Input: part model. Units: mm. Frame: model coordinates. A direction names the side the tool comes from. Give positions to 0.01 mm unless a question says otherwise; leave off trailing zeros. Loops run counter-clockwise (first coordinate to the right, second up) from the corner with the lowest first, then second, coordinate; pieces in that order, holes last. Notation, with made-up numbers: M 11,80.25 L 29,80.25 A29 ccw 29,107.25 Z; hole C -30,-29 d11. An arc over 180 degrees is marked long. Use a Markdown table: item, result. Add a question column.
from build123d import *

# Parameters (mm, degrees)
F1_DEPTH  = 12.7
F2_W      = 12.7
F2_H      = 12.7
F3_DEPTH  = 25.4
F5_DEPTH  = 12.7
F6_R      = 9.525
F7_DEPTH  = 6.35
F7_FACE_R = 9.525
F8_DEPTH  = 19.05
F9_R      = 6.35
F10_DEPTH = 25.4


with BuildPart() as f1:
    # F0 (on Right) → F1 (new body)
    with BuildSketch(Plane.YZ):
        Polygon((0, 19.05), (0, 0), (25.4, 0), (25.4, 19.05), (19.05, 25.4), (6.35, 25.4), align=None)
    extrude(amount=F1_DEPTH)

    # F2 (on face) → F3 (join)
    with BuildSketch(Plane.YZ.offset(12.7)):
        with Locations((12.7, 12.7)):
            Rectangle(F2_W, F2_H)
    extrude(amount=F3_DEPTH)

    # F4 (on face) → F5 (cut)
    with BuildSketch(Plane.XZ.offset(-6.35)):
        with BuildLine():
            Line((38.1, 6.35), (38.1, 19.05))
            Line((38.1, 19.05), (25.4, 19.05))
            ThreePointArc((25.4, 19.05), (22.974516, 12.7), (25.4, 6.35))
            Line((25.4, 6.35), (38.1, 6.35))
        make_face()
    extrude(amount=-F5_DEPTH, mode=Mode.SUBTRACT)



with BuildPart() as f7:
    # F6 (on face) → F7 (new body)
    with BuildSketch(Plane.XZ.offset(-6.35)):
        with Locations((32.499516, 12.7)):
            Circle(F6_R)
    extrude(amount=F7_DEPTH)


with BuildPart() as f1_1:
    add(f1.part)

    add(f7.part)  # F8 merges F7
    # F7_face (on face) → F8 (join)
    with BuildSketch(Plane(origin=(32.499516, 6.35, 12.7), x_dir=(1, 0, 0), z_dir=(0, 1, 0))):
        Circle(F7_FACE_R)
    extrude(amount=F8_DEPTH)

    # F9 (on face) → F10 (cut)
    with BuildSketch(Plane(origin=(0, 25.4, 0), x_dir=(-1, 0, 0), z_dir=(0, 1, 0))):
        with Locations((-32.499516, 12.7)):
            Circle(F9_R)
    extrude(amount=-F10_DEPTH, mode=Mode.SUBTRACT)


solid = f1_1.part
1) Section query A-A, the plane z = 12.7. Return the cut outline in (x, y), and give its area (3 significant figures).
2) Pull-direction query (X, two-part tool) for faces 1 (the flat face through (6.26, 22.27, 22.18)), 2 (the flat face through (0, 13, 13)), 3 (the cylindrical face through (41.585, 12.522, 9.839)); classes: pulls with the +X half, pulls with the -X half, needs draft (parallel to the pull), parting line crosses it, or undercut.
3) Section query B-B, the plane y = 24. Return the cut outline in (x, z) (3 decimals).
4) Ray query, line 1 (X direction, y = 20, z = 12.25); line 2 (Y direction, x = 19.5, z = 9). Return the intervals inside material, ascending. Write a range as [from, to].
5) Section query C-C, the plane x = 34.5. Return the cut outline in (y, z), and give its area (3 significant figures).
6) Section query D-D, the plane y = 8.75. Return the cut outline in (x, z) (3 decimals), and give its area (3 significant figures).
7) Contact query for flat-ended pins moving along their axis: P1, Ø8, axis at x = 18, z = 6.5, coming from the -Y side; P2, Ø6, axis at y = 3, z = 22, coming from the +X side; P3, Ø3, axis at x = 14.5, z = 3.5, coming from the -Y side; P4, Ø5, axis at x = 32, y = 18, coming from the -Z side (3 decimals). Output: stop coordinate, or through.
8) Reachability of faces 4 (the flat face through (19, 13, 19.05)), 5 (the flat face through (6.26, 3.22, 22.27)), 6 (the flat face through (12.7, 13, 4)), 7 (the flat face through (19, 13, 6.35)) from +Z, -Z, +X, -X, +Y, -Y: full face, straight path, thin tool, end or side. Return the list, or none.
Entries:
| question | item | result |
|---|---|---|
| 1 | outline | M 0,0 L 12.7,0 L 12.7,6.35 L 22.97,6.35 L 22.97,0 L 26.15,0 L 26.15,25.4 L 22.97,25.4 L 22.97,19.05 L 12.7,19.05 L 12.7,25.4 L 0,25.4 Z; M 38.85,0 L 42.02,0 L 42.02,25.4 L 38.85,25.4 Z |
| 1 | area | 614 mm² |
| 2 | face 1 | needs draft |
| 2 | face 2 | pulls with the -X half |
| 2 | face 3 | undercut |
| 3 | outline | M 0,0 L 12.7,0 L 12.7,20.45 L 0,20.45 Z; C 32.5,12.7 d19.05; hole C 32.5,12.7 d12.7 |
| 4 | line 1 | x = [0, 12.7], [22.99, 26.17], [38.83, 42.01] |
| 4 | line 2 | y = [6.35, 19.05] |
| 5 | outline | M 0,3.39 L 25.4,3.39 L 25.4,6.67 L 0,6.67 Z; M 0,18.73 L 25.4,18.73 L 25.4,22.01 L 0,22.01 Z |
| 5 | area | 167 mm² |
| 6 | outline | M 0,0 L 12.7,0 L 12.7,6.35 L 25.4,6.35 A9.525 ccw long 25.4,19.05 L 12.7,19.05 L 12.7,25.4 L 0,25.4 Z; hole C 32.5,12.7 d12.7 |
| 6 | area | 621 mm² |
| 7 | P1 | stops at y = 6.35 |
| 7 | P2 | stops at x = 39.64 |
| 7 | P3 | passes through |
| 7 | P4 | stops at z = 3.175 |
| 8 | face 4 | +Z, +Y, -Y |
| 8 | face 5 | +Z, -X, -Y |
| 8 | face 6 | none |
| 8 | face 7 | -Z, +Y, -Y |
